```python
from build123d import *

# Parameters (mm, degrees)
EXTRUDE_1_DEPTH     = 100
CUT_EXTRUDE_1_DEPTH = 101
SKETCH_3_OUTSIDE_W  = 207.148
SKETCH_3_OUTSIDE_H  = 407.148
SKETCH_3_OUTSIDE_R  = 21.770153001
CUT_EXTRUDE_2_DEPTH = 421


with BuildPart() as part:
    # Эскиз1 → Бобышка-Вытянуть1 (new body)
    with BuildSketch(Plane.XY):
        with BuildLine():
            Line((-210, 0), (210, 0))
            Line((210, 0), (210, 220))
            ThreePointArc((210, 220), (186.568542495, 276.568542495), (130, 300))
            Line((130, 300), (-130, 300))
            ThreePointArc((-130, 300), (-186.568542495, 276.568542495), (-210, 220))
            Line((-210, 220), (-210, 0))
        make_face()
    extrude(amount=EXTRUDE_1_DEPTH)

    # Эскиз2 → Вырез-Вытянуть1 (cut, through all)
    with BuildSketch(Plane.XY.offset(100)):
        with BuildLine():
            Line((-180, 0), (180, 0))
            Line((180, 0), (180, 200))
            ThreePointArc((180, 200), (162.426406871, 242.426406871), (120, 260))
            Line((120, 260), (-120, 260))
            ThreePointArc((-120, 260), (-162.426406871, 242.426406871), (-180, 200))
            Line((-180, 200), (-180, 0))
        make_face()
    extrude(amount=-CUT_EXTRUDE_1_DEPTH, mode=Mode.SUBTRACT)

    # Эскиз3 outside → Вырез-Вытянуть2 (cut, through all)
    with BuildSketch(Plane(origin=(210, 0, 0), x_dir=(0, 0, -1), z_dir=(1, 0, 0))):
        with Locations((-50, 150)):
            Rectangle(SKETCH_3_OUTSIDE_W, SKETCH_3_OUTSIDE_H)
        with BuildLine():
            Line((-78.46975089, 299.947886103), (-21.53024911, 300))
            Line((-21.53024911, 300), (-21.53024911, 91.103202847))
            ThreePointArc((-21.53024911, 91.103202847), (-50, 0), (-78.46975089, 91.103202847))
            Line((-78.46975089, 91.103202847), (-78.46975089, 299.947886103))
        make_face(mode=Mode.SUBTRACT)
        with Locations((-50, 50)):
            Circle(SKETCH_3_OUTSIDE_R)
    extrude(amount=-CUT_EXTRUDE_2_DEPTH, mode=Mode.SUBTRACT)


solid = part.part
```
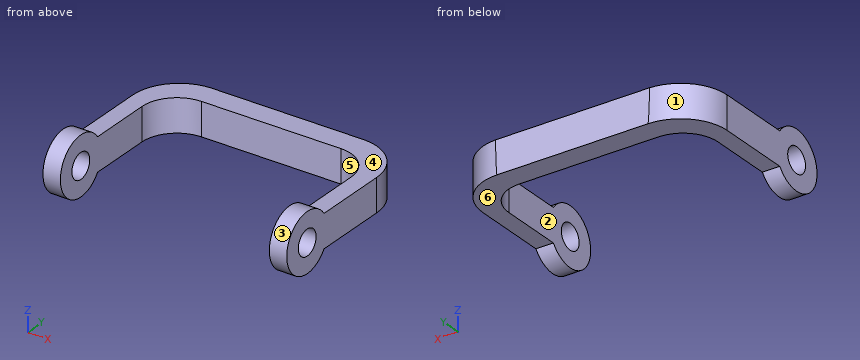
The listing builds one solid part. Answer for the finished solid, in the listing's coordinates (mm). Face numbers are marked on the shaded views. A direction names the side the tool comes from. Coordinates: 2 decimals unless noted, no trailing zeros. Write each loop counter-clockwise with the first axis right and the second up, starting at its lowest first coordinate (ties: lowest second). Pieces come first, ordered by that corner, then holes. Notation, with made-up numbers: M 23,79 L 57,79 A25 cw 57,118 Z; hole C -2.5,-21 d6. An arc over 180 degrees is marked long. Use a Markdown table: item, result. Add a question column.
1. Given P1, Ø4, axis at y = 51, z = 32, coming from the +X side; P2, Ø1, axis at x = -92.5, z = 33, coming from the +Y side; P3, Ø1.5, axis at y = 236.5, z = 64.5, coming from the +X side; P4, Ø5, axis at x = 119, z = 38, coming from the -Y side, each flat-ended and moving along its own axis, determine where each tip first touches the part or whether it passes through.
2. For a pull along X with two mould halves and no side action, classify the marked faces 1, 2 and 3 as +X half, -X half, draft (parallel to the pull), parting line (faces both ways), or undercut.
3. Which of the six approach directions +Z, -Z, +X, -X, +Y, -Y give full straight-line access (tool end or side, diameter ignored) to the marked faces 4, 5 and 6?
4. Section B-B (z = 59.5) is taken. Give the vertices of the cut face in (x, y).
5. Section D-D (x = 52.5) is taken. Give the vertices of the cut face in (y, z), plus the area to 3 significant figures.
6. Section C-C (y = 238) is taken. Give the vertices of the cut face in (x, z), plus the area to 3 significant figures.
7. Straight lines are drawn through the part: line 1 along X through (y, z) = (37, 7.5); line 2 along Y through (x, z) = (20.5, 25); line 3 along Y through (x, z) = (-200, 50). For each, find the intervals that lie inside material, in ascending order. Write a range as [from, to].
8. Section A-A (y = 50) is taken. Give the vertices of the cut face in (x, z), plus the area to 3 significant figures.
Data:
| question | item | result |
|---|---|---|
| 1 | P1 | passes through |
| 1 | P2 | stops at y = 299.99 |
| 1 | P3 | stops at x = 208.43 |
| 1 | P4 | stops at y = 259.98 |
| 2 | face 1 | -X half |
| 2 | face 2 | undercut |
| 2 | face 3 | draft |
| 3 | face 4 | +Z, +X, -X, +Y |
| 3 | face 5 | +Z, -Z, -Y |
| 3 | face 6 | -Z, +X, -X, +Y |
| 4 | outline | M -210,0.91 L -180,0.91 L -180,30.41 L -210,30.41 Z; M -210,69.59 L -180,69.59 L -180,200 A60 cw -120,260 L 120,260 A60 cw 180,200 L 180,69.59 L 210,69.59 L 210,220 A80 ccw 132.36,299.97 L -132.36,299.97 A80 ccw -210,220 Z; M 180,0.91 L 210,0.91 L 210,30.41 L 180,30.41 Z |
| 5 | outline | M 260,21.53 L 300,21.53 L 299.95,78.47 L 260,78.47 Z |
| 5 | area | 2,280 mm2 |
| 6 | outline | M -207.95,21.53 L -166.43,21.53 L -166.43,78.47 L -207.95,78.47 Z; M 166.43,21.53 L 207.95,21.53 L 207.95,78.47 L 166.43,78.47 Z |
| 6 | area | 4,730 mm2 |
| 7 | line 1 | x = [-210, -180], [180, 210] |
| 7 | line 2 | y = [260, 300] |
| 7 | line 3 | y = [0, 28.23], [71.77, 258.73] |
| 8 | outline | M -210,0 L -180,0 L -180,28.23 L -210,28.23 Z; M -210,71.77 L -180,71.77 L -180,100 L -210,100 Z; M 180,0 L 210,0 L 210,28.23 L 180,28.23 Z; M 180,71.77 L 210,71.77 L 210,100 L 180,100 Z |
| 8 | area | 3,390 mm2 |
